The model under review builds one solid part; all positions refer to its coordinate system, in mm. A direction names the side the tool comes from. Round coordinates to 2 decimals unless told otherwise and drop trailing zeros. Order: outer loops, then holes, each group sorted by start corner. A loop starts at its lowest first (then second) coordinate and runs counter-clockwise, first axis right, second up.
Autodesk Inventor part; units mm, degrees
ref_plane "YZ Plane" through (0, 0, 0) normal (1, 0, 0) x (0, 1, 0)
ref_plane "XZ Plane" through (0, 0, 0) normal (0, 1, 0) x (-1, 0, 0)
ref_plane "XY Plane" through (0, 0, 0) normal (0, 0, 1) x (1, 0, 0)
sketch "Sketch1" plane through (0, 0, 0) normal (0, 1, 0) x (-1, 0, 0)
  line L0 (16, 3) -> (-16, 3)
  line L1 (-16, 3) -> (-16, -3)
  line L2 (-16, -3) -> (16, -3)
  line L3 (16, -3) -> (16, 3)
  line L4 (16, 3) -> (-16, -3) construction
  line L5 (-16, 3) -> (16, -3) construction
  point P0 (0, 0)
  dimension "POST_THICKNESS" = 6
  dimension "POST_WIDTH" = 32
extrude "Extrusion1" add sketch "Sketch1" along normal blind 73.912
sketch "Sketch5" plane through (16, 73.912, -3) normal (0, 0, -1) x (-1, 0, 0)
  line L0 (0, 0) -> (32, 0)
  line L1 (16.088, 0) -> (0, -16.088)
  line L2 (0, -73.912) -> (0, 0)
  circle A0 centre (6.088, -10) radius 1.75
  circle A1 centre (9.6235, -6.4645) radius 1
  circle A2 centre (2.5525, -13.5355) radius 1
  line L3 (32.1913, -64.8447) -> (19.6606, -77.3754)
  circle A3 centre (29.4475, -67.5885) radius 1
  circle A4 centre (22.3765, -74.6595) radius 1
  line L4 (32, -73.912) -> (32, 0)
  circle A5 centre (25.912, -71.124) radius 1.75
  line L5 (0, -73.912) -> (32, -73.912)
  point P0 (16, -73.912)
  point P1 (0, -58)
  point P2 (32, -58)
  dimension "d33" = 45
  dimension "d35" = 0
  dimension "d36" = 5
  dimension "d37" = 5
  dimension "d38" = 45
  dimension "d39" = 9.9999
  dimension "d42" = 0
  dimension "d43" = 5
  dimension "d44" = 2
  dimension "d45" = 2
  dimension "d46" = 2
  dimension "d47" = 2
  dimension "BOTTOM_MIRROR_HOLE" = 2.788
  dimension "TOP_MIRROR_HOLE" = 63.912
  dimension "d90" = 9.912
  dimension "d91" = 9.912
  dimension "d92" = 3.5
  dimension "d93" = 3.5
extrude "Extrusion3" cut sketch "Sketch5" against normal blind 3 contours A1 L1 | L1 A1 | A2 L1 | L1 A2 | L5 A4 L3 | A4 L5 | A3 L3 | L3 A3 | L3 A4 picked at (22.0928, -74.8345)
sketch "Sketch6" plane through (16, 0, -3) normal (0, 0, -1) x (-1, 0, 0)
  line L0 (0, 0) -> (0, 73.912)
  line L1 (0, 0) -> (32, 0)
  line L2 (0, 2) -> (32, 2)
  line L3 (32, 2) -> (32, 0)
  line L4 (32, 0) -> (0, 0)
  line L5 (0, 0) -> (0, 2)
  point P0 (16, 0)
  dimension "BASE_HEIGHT" = 2
extrude "Extrusion4" [suppressed]
sketch "Sketch7" plane through (-16, 2, -3) normal (0, 1, 0) x (1, 0, 0)
  line L0 (0, 35) -> (32, 35)
  line L1 (0, 0) -> (0, 35)
  line L2 (32, 0) -> (32, 35)
  point P0 (16, -3)
  point P1 (26, 29)
  point P2 (6, 29)
  dimension "d60" = 6
  dimension "d61" = 6
  dimension "d62" = 6
  dimension "d63" = 0
hole "Hole3" [suppressed]
sketch "Sketch8" plane through (16, 73.912, -3) normal (0, 0, -1) x (-1, 0, 0)
  line L0 (0, 0) -> (32, 0)
  line L1 (12.088, 0) -> (0, -12.088)
  line L2 (0, -60) -> (0, 0)
  circle A0 centre (6.088, -6) radius 1.651
  circle A1 centre (9.6235, -2.4645) radius 1
  circle A2 centre (2.5525, -9.5355) radius 1
  line L3 (32.1913, -28.7207) -> (19.6606, -41.2514)
  circle A3 centre (29.4475, -31.4645) radius 1
  circle A4 centre (22.3765, -38.5355) radius 1
  line L4 (32, -60) -> (32, 0)
  circle A5 centre (25.912, -35) radius 1.651
  point P0 (16, -73.912)
  point P1 (16, -60)
  point P2 (0, -58)
  point P3 (32, -58)
  dimension "d64" = 45
  dimension "d65" = 0
  dimension "d66" = 5
  dimension "d67" = 5
  dimension "d68" = 45
  dimension "d69" = 9.9999
  dimension "d70" = 0
  dimension "d71" = 5
  dimension "d72" = 2
  dimension "d73" = 2
  dimension "d74" = 2
  dimension "d75" = 2
hole "Hole4" [suppressed]
chamfer "Chamfer1" distance 2 angle 45 2 edges at (-16, 73.912, 0) (16, 73.912, 0)
hole "Hole5" at (9.912, 63.912, -3) at (-9.912, 2.788, -3) direction (0, 0, 1) diameter 4.496 depth 5 tip angle 118
sketch "Sketch10" plane through (0, 0, 0) normal (0, -1, 0) x (1, 0, 0)
  line L0 (14, 3) -> (16, 3)
  line L1 (-14, -3) -> (-16, -3)
  line L2 (16, 3) -> (-16, 3)
  line L3 (-16, 3) -> (-16, -3)
  line L4 (-16, -3) -> (16, -3)
  line L5 (16, -3) -> (16, 3)
  point P0 (0, 0)
extrude "Extrusion6" add sketch "Sketch10" along normal blind 18
sketch "Sketch11" plane through (0, -18, 0) normal (0, -1, 0) x (1, 0, 0)
  line L0 (16, 25) -> (-16, 25)
  line L1 (-16, 25) -> (-16, -38)
  line L2 (-16, -38) -> (16, -38)
  line L3 (16, -38) -> (16, 25)
  line L4 (-16, 25) -> (16, 25)
  line L5 (16, 25) -> (16, 15)
  line L6 (16, 15) -> (-16, 15)
  line L7 (-16, 15) -> (-16, 25)
  line L8 (16, -3) -> (-16, -3)
  point P0 (0, 0)
  point P1 (-16, 15)
  dimension "d107" = 32
  dimension "d124" = 10
  dimension "d125" = 35
extrude "Extrusion7" add sketch "Sketch11" against normal blind 5 contours L3 L8 L1 L6 | L3 L2 L1 L8
sketch "Sketch12" plane through (0, -13, 0) normal (0, 1, 0) x (1, 0, 0)
  point P0 (0, 0)
  point P1 (-10, 32)
  point P2 (10, 32)
  point P3 (-10, -10)
  point P4 (10, -10)
  dimension "d116" = 10
  dimension "d117" = 10
  dimension "d118" = 32
  dimension "d119" = 32
  dimension "d120" = 10
  dimension "d121" = 10
  dimension "d122" = 20
  dimension "d123" = 10
hole "Hole6" at (-10, -13, -32) at (10, -13, -32) at (-10, -13, 10) at (10, -13, 10) direction (0, -1, 0) diameter 3.302 depth 8
sketch "Sketch14" plane through (0, -13, 0) normal (0, 1, 0) x (1, 0, 0)
  line L0 (-16, -15) -> (-16, 38)
  line L1 (-16, 27) -> (-12.9595, 27)
  line L2 (-10.9595, 25) -> (-10.9595, 23)
  line L3 (-12.9595, 21) -> (-16, 21)
  line L4 (-16, 21) -> (-16, 27)
  line L5 (14, 3) -> (-14, 3)
  arc A0 (-12.9595, 21) -> (-10.9595, 23) centre (-12.9595, 23) ccw
  arc A1 (-10.9595, 25) -> (-12.9595, 27) centre (-12.9595, 25) ccw
  point P0 (0, 0)
  point P1 (-10.9595, 21)
  point P2 (-10.9595, 27)
  dimension "d127" = 6
  dimension "d128" = 18
  dimension "d131" = 2
extrude "Extrusion8" cut sketch "Sketch14" against normal blind 10
extrude "Extrusion9" cut sketch "Sketch5" against normal blind 3 contours L5 A4 L3 | A4 L5 | L3 A4 picked at (22.0928, -74.8345)
equation "\"BOTTOM_MIRROR_HOLE\" = GROUND_BEAM_HEIGHT - POLARIS_HOLE_TO_MIRROR_HEIGHT"
equation "\"TOP_MIRROR_HOLE\" = LASER_BEAM_HEIGHT + POLARIS_HOLE_TO_MIRROR_HEIGHT"
equation "\"WING_SIZE\" = 8"
equation "\"POLARIS_HOLE_TO_MIRROR_HEIGHT\" = 9.912"
properties part number "L periscope"
(1) Draft analysis for pull direction Y (two halves, no side actions). For faces 1 (the flat face through (6, 67, 0)), 2 (the flat face through (0, -16, 15)), 3 (the flat face through (0, -13, 9)), state which applies: pulls with the +Y half, pulls with the -Y half, needs draft (parallel to the pull), parting line crosses it, or undercut.
Data:
face 1: undercut
face 2: needs draft
face 3: pulls with the +Y half
(2) Consider section B-B (x = -2). Write out the cut boundary in (y, z).
Data:
outline: (-18, -38) - (-13, -38) - (-13, -3) - (73.91, -3) - (73.91, 3) - (-13, 3) - (-13, 15) - (-18, 15) - close
(3) To check wall thickness, follow probe 1 along Z at (x, y) = (-10, -14); probe 2 along X at (y, z) = (-16.8, -32); probe 3 along Y at (x, z) = (12, -27.5). State the ranges of each line that lie inside material, in increasing order.
Data:
probe 1: z = -38 to -33.65, -30.35 to 8.35, 11.65 to 15
probe 2: x = -16 to -11.65, -8.35 to 8.35, 11.65 to 16
probe 3: y = -18 to -13
(4) Consider section D-D (z = -17). Write out the cut boundary in (x, y).
Data:
outline: (-16, -18) - (16, -18) - (16, -13) - (-16, -13) - close
(5) Consider section C-C (y = 25). Write out the cut boundary in (x, z).
Data:
outline: (-16, -3) - (16, -3) - (16, 3) - (-16, 3) - close
(6) Consider section A-A (z = 10). Write out the cut boundary in (x, y).
Data:
outline: (-16, -18) - (-11.65, -18) - (-11.65, -13) - (-16, -13) - close; (-8.35, -18) - (8.35, -18) - (8.35, -13) - (-8.35, -13) - close; (11.65, -18) - (16, -18) - (16, -13) - (11.65, -13) - close
(7) Insertion check: pin 1 (1 mm diameter, centred on x = 13, y = 60, fed in from -Z); pin 2 (1 mm diameter, centred on x = -12.5, z = -7, fed in from +Y); pin 3 (4 mm diameter, centred on x = -8, z = -4, fed in from +Y); pin 4 (0.6 mm diameter, centred on x = -6.5, y = -1, fed in from -Z). Each pin has a flat end and moves straight along its axis. Give the tip position at first contact, or say it passes through.
Data:
pin 1: stops at z = -3
pin 2: stops at y = -13
pin 3: stops at y = 73.91
pin 4: stops at z = 0
(8) For faces 4 (the flat face through (0, 31, 3)), 5 (the cylindrical face through (-11.56, -15.46, -21.57)), 6 (the cylindrical face through (-12.65, 5.72, -1.52)), 7 (the flat face through (0, -16, -38)), list the 3-axis set-ups (+Z, -Z, +X, -X, +Y, -Y) from which the entire face can be reached by the end or side of a thin tool; tool diameter is ignored.
Data:
face 4: +Z, +X, -X, +Y
face 5: -X, +Y, -Y
face 6: -Z
face 7: -Z, +X, -X, +Y, -Y
